Could you check a few things on this model? Use its own coordinates, in mm. Face numbers are marked on the shaded views. A direction names the side the tool comes from. Round coordinates to 2 decimals unless told otherwise and drop trailing zeros. Write each loop counter-clockwise with the first axis right and the second up, starting at its lowest first coordinate (ties: lowest second). Pieces come first, ordered by that corner, then holes. Notation, with made-up numbers: (2.5, 63.5) -> (35.5, 63.5) arc R8 cw to (35.5, 75.5) -> close; hole circle Ø5 at (34, 81). An arc over 180 degrees is marked (long way). Return JSON: item names as keys, results as strings.
from build123d import *

# Parameters (mm, degrees)
F0_W     = 42
F0_H     = 42
F1_DEPTH = 34
F2_R     = 11
F3_DEPTH = 2
F4_R     = 2.5
F5_DEPTH = 20
F6_SIZE  = 5


with BuildPart() as f1:
    # F0 (on Top) → F1 (new body)
    with BuildSketch(Plane.XY):
        Rectangle(F0_W, F0_H)
    extrude(amount=F1_DEPTH)

    # F2 (on face) → F3 (join)
    with BuildSketch(Plane.XY.offset(34)):
        Circle(F2_R)
    extrude(amount=F3_DEPTH)

    # F4 (on face) → F5 (join)
    with BuildSketch(Plane.XY.offset(36)):
        Circle(F4_R)
    extrude(amount=F5_DEPTH)

    # F6
    f6_edges = [f1.edges().sort_by_distance(p)[0] for p in [
        (-21, 21, 17),
        (21, 21, 17),
        (21, -21, 17),
        (-21, -21, 17),
    ]]
    chamfer(f6_edges, length=F6_SIZE)


solid = f1.part
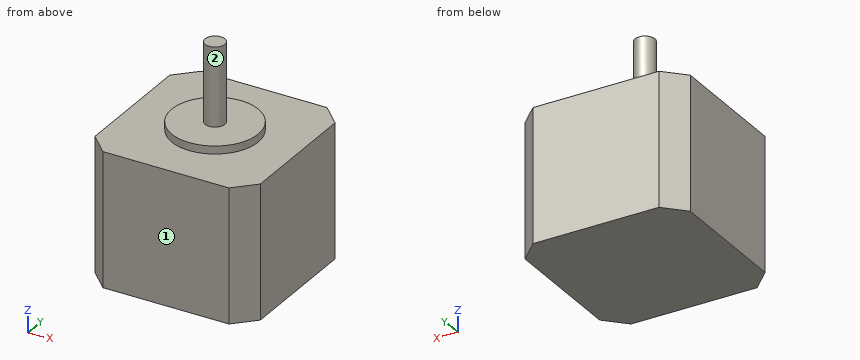
1) If I drill on probe 1 along Z at (x, y) = (13, -7); probe 2 along Z at (x, y) = (2.5, 9); probe 3 along Y at (x, z) = (-0.5, 44.5), over which ranges is the centre line in solid material (lowest first)? Write a range as [from, to].
Return value:
{"probe 1": "[0, 34]", "probe 2": "[0, 36]", "probe 3": "[-2.45, 2.45]"}
2) I want a section at C-C, the plane z = 8. Please give me the cut outline in (x, y).
Return value:
{"outline": "(-21, -16) -> (-16, -21) -> (16, -21) -> (21, -16) -> (21, 16) -> (16, 21) -> (-16, 21) -> (-21, 16) -> close"}
3) Will these pins go through, and if not, where does the flat tip stop? pin 1 Ø12 at (x, y) = (9.5, -4.5) entering from -Z; pin 2 Ø10 at (x, y) = (-10, -3.5) entering from +Z; pin 3 Ø5 at (x, y) = (15, 4.5) entering from +Z.
Return value:
{"pin 1": "z = 0", "pin 2": "z = 36", "pin 3": "z = 34"}
4) For the marked faces 1 and 2, which set-ups out of +Z, -Z, +X, -X, +Y, -Y let a thin tool reach every point of the face, with its end or its side?
Return value:
{"face 1": "+Z, -Z, +X, -X, -Y", "face 2": "+Z"}
5) I want a section at A-A, the plane y = 0. Please give me the cut outline in (x, z).
Return value:
{"outline": "(-21, 0) -> (21, 0) -> (21, 34) -> (11, 34) -> (11, 36) -> (2.5, 36) -> (2.5, 56) -> (-2.5, 56) -> (-2.5, 36) -> (-11, 36) -> (-11, 34) -> (-21, 34) -> close"}
6) I want a section at D-D, the plane x = -8. Please give me the cut outline in (y, z), and give its area (3 significant figures).
Return value:
{"outline": "(-21, 0) -> (21, 0) -> (21, 34) -> (7.55, 34) -> (7.55, 36) -> (-7.55, 36) -> (-7.55, 34) -> (-21, 34) -> close", "area": "1,460 mm²"}
